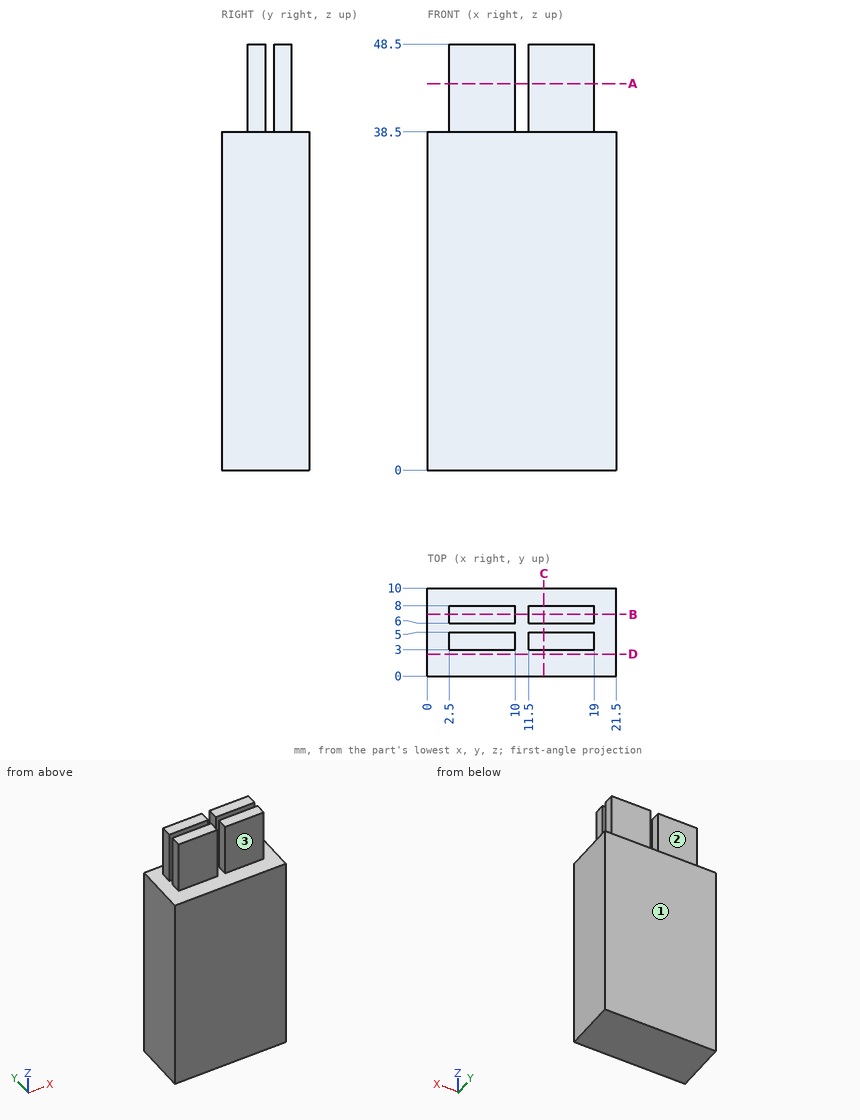
The drawing under review shows one solid part. Ordinate dimensions are in mm from its lowest x, y, z. A direction names the side the tool comes from. Give positions to 0.01 mm unless a question says otherwise; leave off trailing zeros. Write each loop counter-clockwise with the first axis right and the second up, starting at its lowest first coordinate (ties: lowest second). Pieces come first, ordered by that corner, then holes. Notation, with made-up numbers: (-2, 31.25) -> (8, 31.25) arc R17 cw to (8, 40.25) -> close; hole circle Ø8 at (49.5, 50). An arc over 180 degrees is marked (long way). Use CSV: the item, a comma, the result in double quotes.
Q1. For P1, Ø1.6, axis at y = 6.5, z = 46, coming from the -X side; P2, Ø1, axis at y = 6.5, z = 41, coming from the +X side; P3, Ø4, axis at x = 15.5, z = 43.5, coming from the +Y side, all flat-tipped, find the tip position at first contact; note any pin that passes through.
Conclusion:
P1,"x = 2.5"
P2,"x = 19"
P3,"y = 8"
Q2. Take a section at C-C, the plane x = 13.25. Write out the cut boundary in (y, z).
Conclusion:
outline,"(0, 0) -> (10, 0) -> (10, 38.5) -> (8, 38.5) -> (8, 48.5) -> (6, 48.5) -> (6, 38.5) -> (5, 38.5) -> (5, 48.5) -> (3, 48.5) -> (3, 38.5) -> (0, 38.5) -> close"
Q3. Take a section at A-A, the plane z = 44. Write out the cut boundary in (x, y), then the cut area to 3 significant figures.
Conclusion:
outline,"(2.5, 3) -> (10, 3) -> (10, 5) -> (2.5, 5) -> close; (2.5, 6) -> (10, 6) -> (10, 8) -> (2.5, 8) -> close; (11.5, 3) -> (19, 3) -> (19, 5) -> (11.5, 5) -> close; (11.5, 6) -> (19, 6) -> (19, 8) -> (11.5, 8) -> close"
area,"60.0 mm2"
Q4. Take a section at D-D, the plane y = 2.5. Write out the cut boundary in (x, z), then the cut area to 3 significant figures.
Conclusion:
outline,"(0, 0) -> (21.5, 0) -> (21.5, 38.5) -> (0, 38.5) -> close"
area,"828 mm2"
Q5. Tool access review of the marked faces 1, 2 and 3: name each direction out of +Z, -Z, +X, -X, +Y, -Y from which nothing blocks a thin tool from reaching the whole face with its end or side.
Conclusion:
face 1,"+Z, -Z, +X, -X, +Y"
face 2,"+Z, +X, -X, +Y"
face 3,"+Z, +X, -X, -Y"
Q6. To check wall thickness, follow probe 1 along X at (y, z) = (6.25, 43); probe 2 along Z at (x, y) = (5.75, 9). State the ranges of each line that lie inside material, in increasing order. Write a range as [from, to].
Conclusion:
probe 1,"[2.5, 10], [11.5, 19]"
probe 2,"[0, 38.5]"
Q7. Take a section at B-B, the plane y = 7. Write out the cut boundary in (x, z).
Conclusion:
outline,"(0, 0) -> (21.5, 0) -> (21.5, 38.5) -> (19, 38.5) -> (19, 48.5) -> (11.5, 48.5) -> (11.5, 38.5) -> (10, 38.5) -> (10, 48.5) -> (2.5, 48.5) -> (2.5, 38.5) -> (0, 38.5) -> close"
